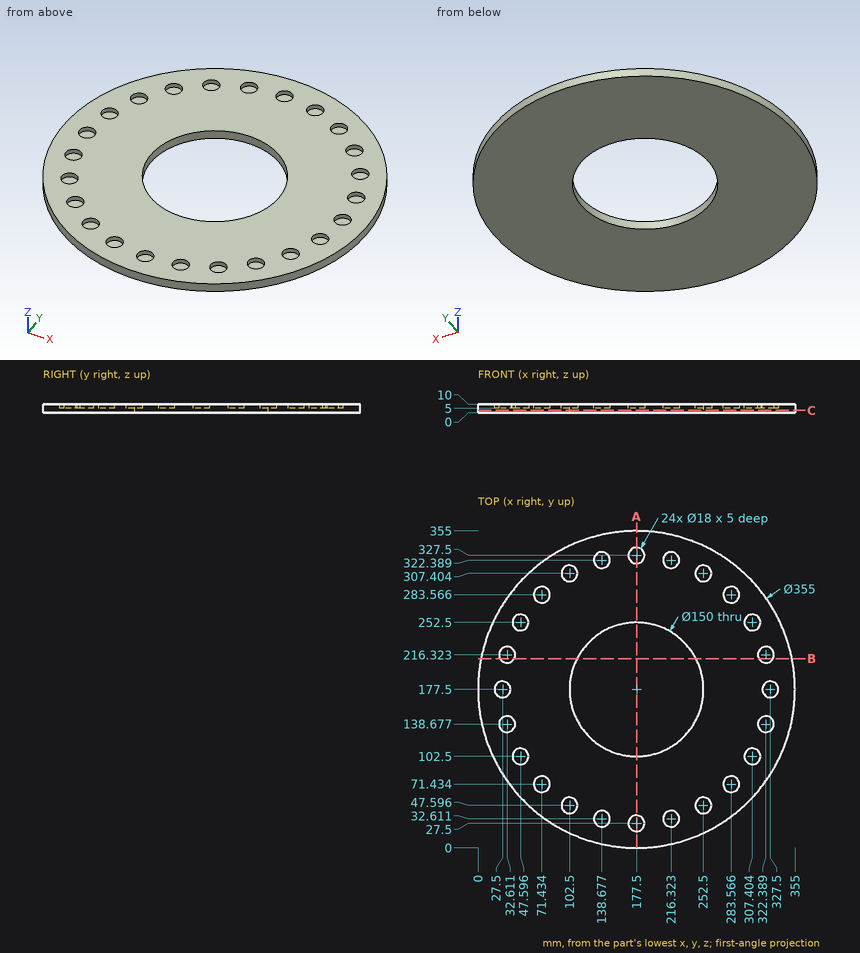
Part print with two shaded views. Sizes in mm from the minimum x, y, z corner. Round coordinates to 2 decimals unless told otherwise and drop trailing zeros. Order: outer loops, then holes, each group sorted by start corner. A loop starts at its lowest first (then second) coordinate and runs counter-clockwise, first axis right, second up. Notation, with made-up numbers: M 78,37.25 L 103,37.25 A15 cw 103,63.25 Z; hole C -6.5,23.25 d2. An arc over 180 degrees is marked long. Answer in a Markdown table with one row per item. Add a question column.
Q1. Cut at B-B on y = 212. Give the cut face in (x, z) (1 decimal), and give its area (3 significant figures).
Q2. Cut at C-C on z = 2.75. Give the cut face in (x, y), and give its area (3 significant figures).
Q3. Pin check, flat tips, straight feed: pin 1 (16 mm diameter, centred on x = 102.5, y = 307.4, fed in from +Z); pin 2 (6 mm diameter, centred on x = 268, z = 8.5, fed in from +Y) (1 decimal); pin 3 (1.5 mm diameter, centred on x = 317, z = 7, fed in from +Y). Stop position of each tip, or through.
Q4. Wall check: L1, parallel to Y at x = 210, z = 6.75 (1 decimal); L2, parallel to X at y = 74, z = 8; L3, parallel to Y at x = 45, z = 9.25. Give the ranges that are in metal, low to high. Write a range as from..to.
Q5. Cut at A-A on x = 177.5. Give the cut face in (y, z), and give its area (3 significant figures).
Established:
| question | item | result |
|---|---|---|
| 1 | outline | M 3.4,0 L 110.9,0 L 110.9,10 L 40.5,10 L 40.5,5 L 24.7,5 L 24.7,10 L 3.4,10 Z; M 244.1,0 L 351.6,0 L 351.6,10 L 330.3,10 L 330.3,5 L 314.5,5 L 314.5,10 L 244.1,10 Z |
| 1 | area | 1,990 mm2 |
| 2 | outline | C 177.5,177.5 d355; hole C 177.5,177.5 d150 |
| 2 | area | 81,300 mm2 |
| 3 | pin 1 | stops at z = 5 |
| 3 | pin 2 | stops at y = 331.9 |
| 3 | pin 3 | stops at y = 288.2 |
| 4 | L1 | y = 3..26.2, 39..109.9, 245.1..316, 328.8..352 |
| 4 | L2 | x = 33.3..62.81, 80.06..274.94, 292.19..321.7 |
| 4 | L3 | y = 59.39..93.88, 111.12..243.88, 261.12..295.61 |
| 5 | outline | M 0,0 L 102.5,0 L 102.5,10 L 36.5,10 L 36.5,5 L 18.5,5 L 18.5,10 L 0,10 Z; M 252.5,0 L 355,0 L 355,10 L 336.5,10 L 336.5,5 L 318.5,5 L 318.5,10 L 252.5,10 Z |
| 5 | area | 1,870 mm2 |
